Can you work these out from the model? Positions are in its coordinate system, mm. Round coordinates to 2 decimals unless told otherwise and drop trailing zeros. Loops run counter-clockwise (first coordinate to the right, second up) from the corner with the lowest first, then second, coordinate; pieces in that order, holes last.
(1) If I drill on line 1 along X through (y, z) = (-19.05, 5.5); line 2 along Y through (x, z) = (1.5, 4); line 3 along Y through (x, z) = (-12, 5), over which ranges is the centre line in solid material (lowest first)?
(2) I want a section at C-C on x = -20.5. Write out the boundary of the cut face in (y, z).
(3) I want a section at A-A on z = 11.25. Write out the boundary of the cut face in (x, y) (3 decimals).
(4) I want a section at B-B on y = -26.5. Write out the boundary of the cut face in (x, z).
from build123d import *

# Parameters (mm, degrees)
F1_DEPTH = 19.05


with BuildPart() as f1:
    # F0 (on Top) → F1 (new body)
    with BuildSketch(Plane.XY):
        with BuildLine():
            ThreePointArc((25.4, -19.05), (-17.960512, -1.089488), (0, -44.45))
            ThreePointArc((0, -44.45), (17.960512, -37.010512), (25.4, -19.05))
        make_face()
        Polygon((-69.85, 69.85), (-69.85, -69.85), (0, -69.85), (69.85, -69.85), (69.85, 69.85), align=None)
        with BuildLine():
            ThreePointArc((3.175, -57.15), (2.245064, -59.395064), (0, -60.325))
            ThreePointArc((0, -60.325), (-3.175, -57.15), (0, -53.975))
            ThreePointArc((0, -53.975), (2.245064, -54.904936), (3.175, -57.15))
        make_face(mode=Mode.SUBTRACT)
        with BuildLine():
            ThreePointArc((25.4, -19.05), (17.960512, -37.010512), (0, -44.45))
            ThreePointArc((0, -44.45), (-17.960512, -1.089488), (25.4, -19.05))
        make_face(mode=Mode.SUBTRACT)
    extrude(amount=F1_DEPTH)


solid = f1.part
Filled sheet:
1. line 1: x = -69.85 to -25.4, 25.4 to 69.85
1. line 2: y = -69.85 to -59.95, -54.35 to -44.41, 6.31 to 69.85
1. line 3: y = -69.85 to -41.44, 3.34 to 69.85
2. outline: (-69.85, 0) - (-34.05, 0) - (-34.05, 19.05) - (-69.85, 19.05) - close; (-4.05, 0) - (69.85, 0) - (69.85, 19.05) - (-4.05, 19.05) - close
3. outline: (-69.85, -69.85) - (69.85, -69.85) - (69.85, 69.85) - (-69.85, 69.85) - close; hole circle Ø50.8 at (0, -19.05); hole circle Ø6.35 at (0, -57.15)
4. outline: (-69.85, 0) - (-24.28, 0) - (-24.28, 19.05) - (-69.85, 19.05) - close; (24.28, 0) - (69.85, 0) - (69.85, 19.05) - (24.28, 19.05) - close
